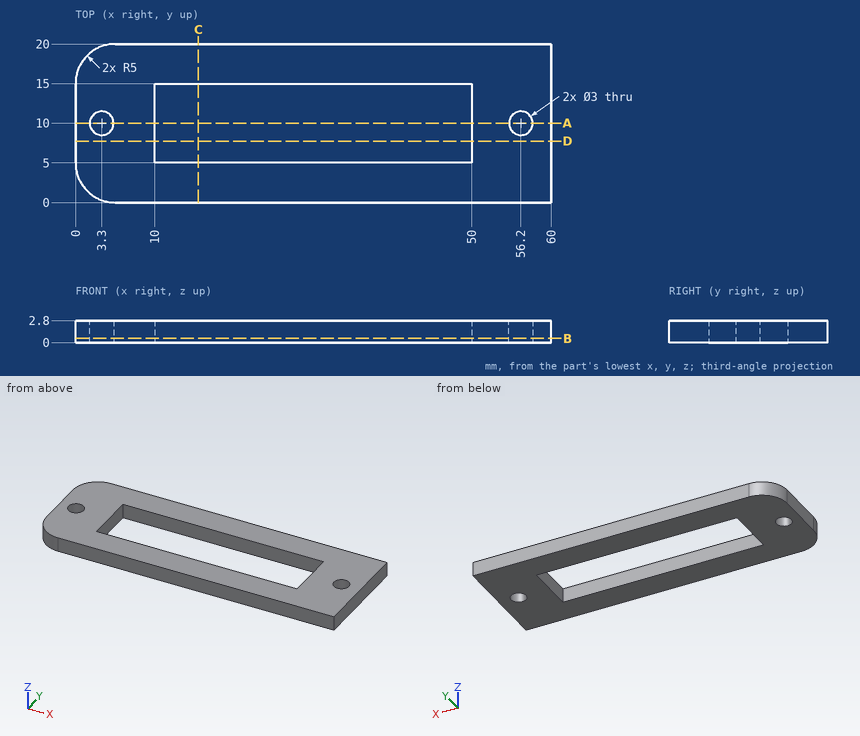
For this review, use the dimensioned drawing (mm, ordinates from the lowest corner) and the shaded views. Coordinates: 2 decimals unless noted, no trailing zeros. Loops run counter-clockwise (first coordinate to the right, second up) from the corner with the lowest first, then second, coordinate; pieces in that order, holes last.
1. Insertion check: P1, Ø2.5, axis at x = 56.2, y = 10, coming from the +Z side. The pin has a flat end and moves straight along its axis. Give the tip position at first contact, or say it passes through.
2. Add section C-C, the plane x = 15.5. Give the boundary of the cut face in (y, z).
3. Add section D-D, the plane y = 7.75. Give the boundary of the cut face in (x, z).
4. Add section A-A, the plane y = 10. Give the boundary of the cut face in (x, z), then the cut area to 3 significant figures.
5. For line 1 (Y direction, x = 56.2, z = 1.3); line 2 (X direction, y = 6.25, z = 0.2); line 3 (Y direction, x = 47, z = 2.3), list the stretches that pass through material, from the lowest coordinate up.
6. Add section B-B, the plane z = 0.55. Give the boundary of the cut face in (x, y), then the cut area to 3 significant figures.
Result:
1. P1: passes through
2. outline: (0, 0) - (5, 0) - (5, 2.8) - (0, 2.8) - close; (15, 0) - (20, 0) - (20, 2.8) - (15, 2.8) - close
3. outline: (0, 0) - (10, 0) - (10, 2.8) - (0, 2.8) - close; (50, 0) - (60, 0) - (60, 2.8) - (50, 2.8) - close
4. outline: (0, 0) - (1.8, 0) - (1.8, 2.8) - (0, 2.8) - close; (4.8, 0) - (10, 0) - (10, 2.8) - (4.8, 2.8) - close; (50, 0) - (54.7, 0) - (54.7, 2.8) - (50, 2.8) - close; (57.7, 0) - (60, 0) - (60, 2.8) - (57.7, 2.8) - close
4. area: 39.2 mm2
5. line 1: y = 0 to 8.5, 11.5 to 20
5. line 2: x = 0 to 10, 50 to 60
5. line 3: y = 0 to 5, 15 to 20
6. outline: (0, 5) arc R5 ccw to (5, 0) - (60, 0) - (60, 20) - (5, 20) arc R5 ccw to (0, 15) - close; hole circle Ø3 at (3.3, 10); hole (10, 5) - (50, 5) - (50, 15) - (10, 15) - close; hole circle Ø3 at (56.2, 10)
6. area: 775 mm2
